Part model, mm, in its own coordinate system. A direction names the side the tool comes from. Give positions to 0.01 mm unless a question says otherwise; leave off trailing zeros. Order: outer loops, then holes, each group sorted by start corner. A loop starts at its lowest first (then second) coordinate and runs counter-clockwise, first axis right, second up.
Autodesk Fusion 360 part; units mm, degrees
sketch "Sketch1" plane through (0, 0, 0) normal (0, 0, 1) x (1, 0, 0)
  line L0 (0.5, 0) -> (30, 0)
  line L1 (30.5, 0.5) -> (30.5, 4)
  line L2 (30, 4.5) -> (0.5, 4.5)
  line L3 (0, 4) -> (0, 0.5)
  arc A0 (0, 0.5) -> (0.5, 0) centre (0.5, 0.5) ccw
  arc A1 (0.5, 4.5) -> (0, 4) centre (0.5, 4) ccw
  arc A2 (30.5, 4) -> (30, 4.5) centre (30, 4) ccw
  arc A3 (30, 0) -> (30.5, 0.5) centre (30, 0.5) ccw
  line L4 (-18.1072, 2.25) -> (79.1072, 2.25) construction
  circle A4 centre (14.4, -1) radius 0.4
  circle A5 centre (-0.3, -1) radius 0.4
  circle A6 centre (7, -1) radius 0.4
  circle A7 centre (21.8, -1) radius 0.4
  circle A8 centre (29.1, -1) radius 0.4
  circle A9 centre (34.1, -1) radius 0.4
  line L5 (-2.117, -1) -> (37.883, -1) construction
  circle A10 centre (34.1, 5.5) radius 0.4
  circle A11 centre (29.1, 5.5) radius 0.4
  circle A12 centre (21.8, 5.5) radius 0.4
  circle A13 centre (14.4, 5.5) radius 0.4
  circle A14 centre (7, 5.5) radius 0.4
  circle A15 centre (-0.3, 5.5) radius 0.4
  line L6 (24, 2.25) -> (37, 2.25) construction
  line L7 (33, 4.7661) -> (33, -0.2339)
  line L8 (-1, 6.9) -> (34.8, 6.9)
  line L9 (35.5, 6.2) -> (35.5, -1.7)
  line L10 (34.8, -2.4) -> (-1, -2.4)
  line L11 (-1.7, -1.7) -> (-1.7, 6.2)
  arc A16 (-1, 6.9) -> (-1.7, 6.2) centre (-1, 6.2) ccw
  arc A17 (-1.7, -1.7) -> (-1, -2.4) centre (-1, -1.7) ccw
  arc A18 (34.8, -2.4) -> (35.5, -1.7) centre (34.8, -1.7) ccw
  arc A19 (35.5, 6.2) -> (34.8, 6.9) centre (34.8, 6.2) ccw
  circle A20 centre (33, 2.2661) radius 1.15
  point P0 (30.5, 0)
  point P1 (0, 4.5)
  point P2 (-1.7, 6.9)
  point P3 (35.5, 6.9)
  point P4 (-1.7, -2.4)
  dimension "d1" = 30.5
  dimension "d2" = 4.5
  dimension "d3" = 0.5
  dimension "d4" = 0.5
  dimension "d5" = 0.5
  dimension "d6" = 0.5
  dimension "d7" = 0.8
  dimension "d8" = 0.8
  dimension "d9" = 0.8
  dimension "d10" = 0.8
  dimension "d11" = 0.8
  dimension "d12" = 0.8
  dimension "d13" = 5
  dimension "d14" = 12.3
  dimension "d15" = 19.7
  dimension "d16" = 27.1
  dimension "d17" = 34.4
  dimension "d18" = 3.6
  dimension "d20" = 5.5
  dimension "d21" = 6.5
  dimension "d22" = 37.2
  dimension "d23" = 9.3
  dimension "d24" = 1.4
  dimension "d25" = 1.4
  dimension "d27" = 1.4
  dimension "d28" = 0.7
  dimension "d29" = 0.7
  dimension "d30" = 0.7
  dimension "d31" = 0.7
  dimension "d32" = 2.5
  dimension "d33" = 2.3
  dimension "d34" = 33.4598
extrude "Extrude1" add sketch "Sketch1" along normal mid plane 1
Item 1: Pull direction Y, two halves, no side cores. Call faces 3 (the face through (-1.7, 2, 0)), 4 (the face through (17, 6.9, 0)), 5 (the face through (17, -2.4, 0)), 6 (the face through (0, 2, 0)): released by +Y, released by -Y, zero draft, split by the parting line, or undercut.
Item 2: Drop a flat-ended pin along its axis: P1, Ø3, axis at x = 17, y = 0.5, coming from the +Z side. Give the stop position or say it passes through.
Item 3: Band-saw the part on A-A on x = 7. List the corners of the cut face in (y, z), plus the area to 3 significant figures.
Item 4: Which spindle directions (+Z, -Z, +X, -X, +Y, -Y) get a long thin tool onto all of the face, cutting with end or side? Do faces 1 (the face through (30.5, 2, 0)), 2 (the face through (35.5, 2, 0)). Say none if no direction does.
Item 5: Band-saw the part on D-D on z = -0.2. Give the number of separate pieces and of enclosed holes in the cut face, plus the area to 3 significant figures.
Item 6: Drill centre lines: probe 1 along Y at (x, z) = (21.8, -0.25); probe 2 along Y at (x, z) = (18, -0.25); probe 3 along X at (y, z) = (4, 0.1). Where is each one in solid material? Low to high.
Item 7: Band-saw the part on B-B on y = 1.75. List the corners of the cut face in (x, z), plus the area to 3 significant figures.
Item 8: Band-saw the part on C-C on x = 26.5. List the corners of the cut face in (y, z), plus the area to 3 significant figures.
Working result:
1. face 3: zero draft
1. face 4: released by +Y
1. face 5: released by -Y
1. face 6: undercut
2. P1: stops at z = 0.5
3. outline: (-2.4, -0.5) - (-1.4, -0.5) - (-1.4, 0.5) - (-2.4, 0.5) - close; (-0.6, -0.5) - (0, -0.5) - (0, 0.5) - (-0.6, 0.5) - close; (4.5, -0.5) - (5.1, -0.5) - (5.1, 0.5) - (4.5, 0.5) - close; (5.9, -0.5) - (6.9, -0.5) - (6.9, 0.5) - (5.9, 0.5) - close
3. area: 3.20 mm2
4. face 1: +Z, -Z
4. face 2: +Z, -Z, +X, +Y, -Y
5. separate pieces: 1
5. enclosed holes: 14
5. area: 198 mm2
6. probe 1: y = -2.4 to -1.4, -0.6 to 0, 4.5 to 5.1, 5.9 to 6.9
6. probe 2: y = -2.4 to 0, 4.5 to 6.9
6. probe 3: x = -1.7 to 0, 30.5 to 35.5
7. outline: (-1.7, -0.5) - (0, -0.5) - (0, 0.5) - (-1.7, 0.5) - close; (30.5, -0.5) - (31.97, -0.5) - (31.97, 0.5) - (30.5, 0.5) - close; (34.03, -0.5) - (35.5, -0.5) - (35.5, 0.5) - (34.03, 0.5) - close
7. area: 4.64 mm2
8. outline: (-2.4, -0.5) - (0, -0.5) - (0, 0.5) - (-2.4, 0.5) - close; (4.5, -0.5) - (6.9, -0.5) - (6.9, 0.5) - (4.5, 0.5) - close
8. area: 4.80 mm2
